CAD build for the part. Positions are in the model's coordinates, mm. Face numbers are marked on the shaded views. Coordinates: 2 decimals unless noted, no trailing zeros. Order: outer loops, then holes, each group sorted by start corner. A loop starts at its lowest first (then second) coordinate and runs counter-clockwise, first axis right, second up. Notation, with made-up numbers: M 26.5,-7 L 85.5,-7 A20 cw 85.5,10 Z; hole C -19.75,3.25 d2. An arc over 180 degrees is marked long. One line per item, written item: value.
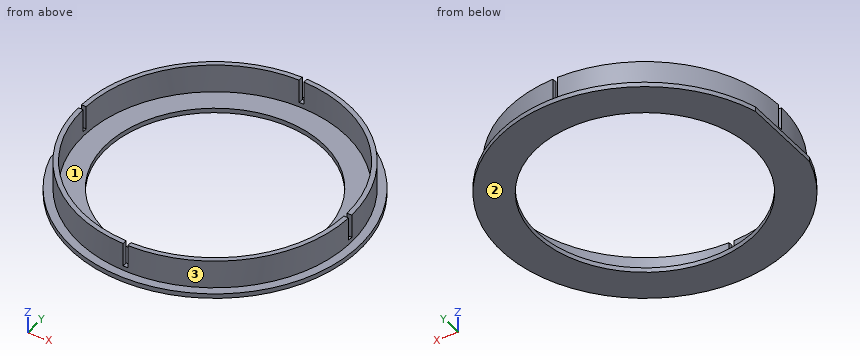
from build123d import *

# Parameters (mm, degrees)
F0_R      = 61
F1_DEPTH  = 2
F2_R      = 57.5
F3_DEPTH  = 12
F4_R      = 46
F5_DEPTH  = 112.4
F6_R      = 55.5
F6_R_2    = 46
F7_DEPTH  = 12
F9_DEPTH  = 25
F10_W     = 130.4447948933
F10_H     = 2
F11_DEPTH = 10
F12_W     = 2
F12_H     = 119
F13_DEPTH = 10


with BuildPart() as f1:
    # F0 (on Top) → F1 (new body)
    with BuildSketch(Plane.XY):
        Circle(F0_R)
    extrude(amount=F1_DEPTH)

    # F2 (on face) → F3 (join)
    with BuildSketch(Plane.XY.offset(2)):
        Circle(F2_R)
    extrude(amount=F3_DEPTH)

    # F4 (on face) → F5 (cut)
    with BuildSketch(Plane.XY.offset(14)):
        Circle(F4_R)
    extrude(amount=-F5_DEPTH, mode=Mode.SUBTRACT)

    # F6 (on face) → F7 (cut)
    with BuildSketch(Plane.XY.offset(14)):
        Circle(F6_R)
        Circle(F6_R_2, mode=Mode.SUBTRACT)
    extrude(amount=-F7_DEPTH, mode=Mode.SUBTRACT)

    # F8 (on face) → F9 (cut)
    with BuildSketch(Plane.XY.offset(2)):
        with BuildLine():
            Line((-58.5, -17.2843860174), (-58.5, 17.2843860174))
            ThreePointArc((-58.5, 17.2843860174), (-61, 0), (-58.5, -17.2843860174))
        make_face()
    extrude(amount=-F9_DEPTH, mode=Mode.SUBTRACT)

    # F10 (on face) → F11 (cut)
    with BuildSketch(Plane.XY.offset(14)):
        Rectangle(F10_W, F10_H)
    extrude(amount=-F11_DEPTH, mode=Mode.SUBTRACT)

    # F12 (on face) → F13 (cut)
    with BuildSketch(Plane.XY.offset(14)):
        Rectangle(F12_W, F12_H)
    extrude(amount=-F13_DEPTH, mode=Mode.SUBTRACT)


solid = f1.part
Q1. Drill centre lines: line 1 along Y through (x, z) = (0, 0.85); line 2 along Z through (x, y) = (-37, 28); line 3 along X through (y, z) = (-35, 3.25). Where is each one in solid material? Low to high.
Recorded:
line 1: y = -61 to -46, 46 to 61
line 2: z = 0 to 2
line 3: x = -45.62 to -43.07, 43.07 to 45.62
Q2. Slice it at A-A (z = 12). List the corners of the cut face in (x, y).
Recorded:
outline: M -57.49,-1 A57.5 ccw -1,-57.49 L -1,-55.49 A55.5 cw -55.49,-1 Z; M -57.49,1 L -55.49,1 A55.5 cw -1,55.49 L -1,57.49 A57.5 ccw Z; M 1,-57.49 A57.5 ccw 57.49,-1 L 55.49,-1 A55.5 cw 1,-55.49 Z; M 1,55.49 A55.5 cw 55.49,1 L 57.49,1 A57.5 ccw 1,57.49 Z
Q3. Slice it at C-C (y = -37). List the corners of the cut face in (x, z).
Recorded:
outline: M -48.5,0 L -27.33,0 L -27.33,2 L -41.37,2 L -41.37,14 L -44.01,14 L -44.01,2 L -48.5,2 Z; M 27.33,0 L 48.5,0 L 48.5,2 L 44.01,2 L 44.01,14 L 41.37,14 L 41.37,2 L 27.33,2 Z
Q4. Pin check, flat tips, straight feed: pin 1 Ø5 at (x, z) = (-12, 9.5) entering from -Y; pin 2 Ø0.6 at (x, y) = (-56.5, -0.5) entering from +Z; pin 3 Ø3 at (x, z) = (-19.5, 6) entering from -Y. Stop position of each tip, or through.
Recorded:
pin 1: stops at y = -56.71
pin 2: stops at z = 4
pin 3: stops at y = -54.61
Q5. Mould opens along X. For the marked faces 1, 2 and 3 say: released by +X, released by -X, zero draft, split by the parting line, or undercut.
Recorded:
face 1: undercut
face 2: zero draft
face 3: split by the parting line
Q6. Slice it at B-B (x = -5.5). List the corners of the cut face in (y, z), plus the area to 3 significant figures.
Recorded:
outline: M -60.75,0 L -45.67,0 L -45.67,2 L -55.23,2 L -55.23,14 L -57.24,14 L -57.24,2 L -60.75,2 Z; M 45.67,0 L 60.75,0 L 60.75,2 L 57.24,2 L 57.24,14 L 55.23,14 L 55.23,2 L 45.67,2 Z
area: 109 mm^2
Q7. Slice it at D-D (x = 51). List the corners of the cut face in (y, z).
Recorded:
outline: M -33.47,0 L 33.47,0 L 33.47,2 L 26.56,2 L 26.56,14 L 21.89,14 L 21.89,2 L -21.89,2 L -21.89,14 L -26.56,14 L -26.56,2 L -33.47,2 Z
